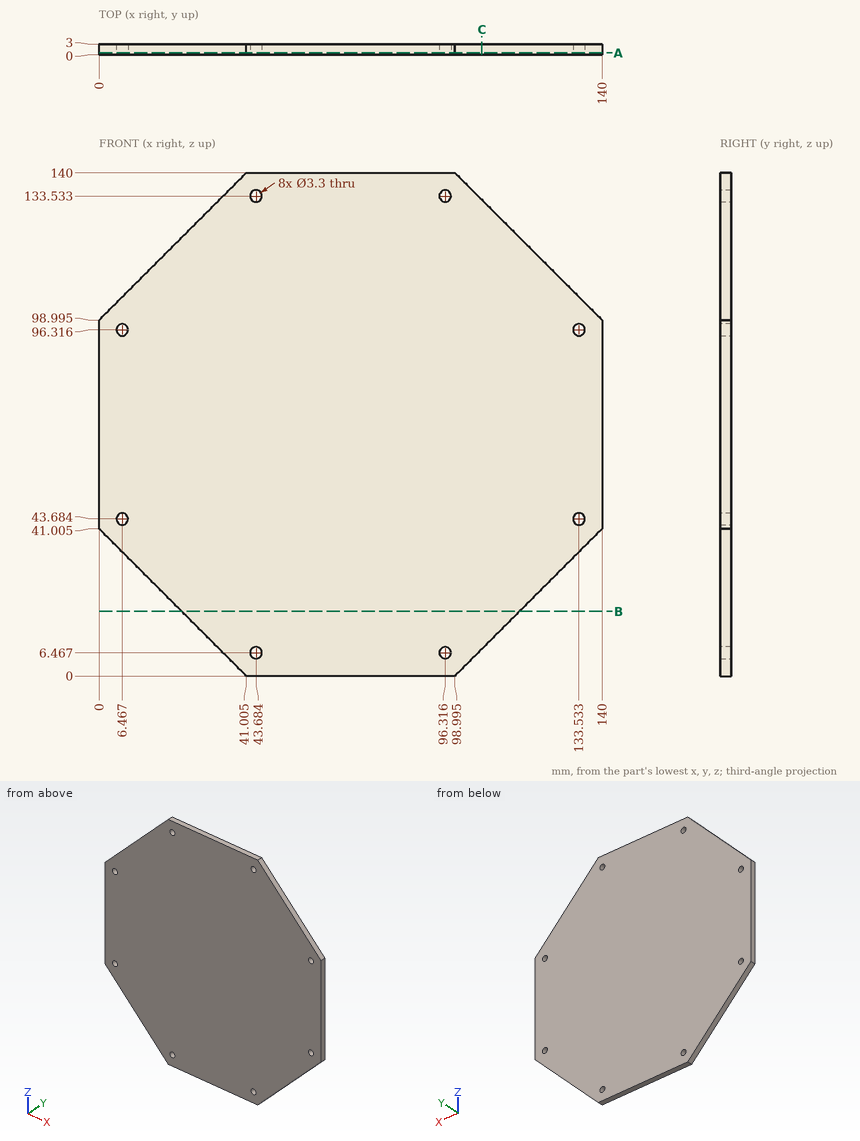
Geometry check sheet. Reference: drawing and pictorial views, mm from the part's lowest x, y, z. Round coordinates to 2 decimals unless told otherwise and drop trailing zeros. Order: outer loops, then holes, each group sorted by start corner. A loop starts at its lowest first (then second) coordinate and runs counter-clockwise, first axis right, second up.
Q1. Scan lines: L1, parallel to Z at x = 133.5, y = 2.5 (1 decimal); L2, parallel to X at y = 2.75, z = 20 (1 decimal); L3, parallel to Z at x = 28, y = 0.8 (1 decimal). Record each from-to range of solid material in increasing order.
Filled sheet:
L1: z = 34.5 to 42, 45.3 to 94.7, 98 to 105.5
L2: x = 21 to 119
L3: z = 13 to 127
Q2. Cross-section at B-B, the plane z = 18. Enter the section's corners in (x, y) (3 decimals).
Filled sheet:
outline: (23.005, 0) - (116.995, 0) - (116.995, 3) - (23.005, 3) - close
Q3. Depth check by flat-ended pin: P1, Ø3, axis at x = 96.32, z = 6.47, coming from the -Y side; P2, Ø1.5, axis at y = 2, z = 125, coming from the +X side (1 decimal). Enter the tip coordinate at first touch or a pass-through.
Filled sheet:
P1: passes through
P2: stops at x = 114.7
Q4. Cross-section at A-A, the plane y = 0.55. Give the number of separate pieces and of enclosed holes in the cut face, plus the area to 3 significant figures.
Filled sheet:
separate pieces: 1
enclosed holes: 8
area: 16,200 mm2
Q5. Cross-section at C-C, the plane x = 106.5. Enter the section's corners in (y, z) (3 decimals).
Filled sheet:
outline: (0, 7.505) - (3, 7.505) - (3, 132.495) - (0, 132.495) - close
